Source: CAD feature listing. Evaluate the final solid. Frame: model axes, mm. Give positions to 0.01 mm unless a question says otherwise; leave off trailing zeros. Order: outer loops, then holes, each group sorted by start corner. A loop starts at its lowest first (then second) coordinate and runs counter-clockwise, first axis right, second up. Notation, with made-up numbers: (24.5, 85.5) -> (71.5, 85.5) arc R20 cw to (71.5, 93.5) -> close; hole circle Ø5 at (-34.5, -15.5). An arc over 180 degrees is marked (long way). Answer in a Markdown table with one row per item.
```python
from build123d import *

# Parameters (mm, degrees)
BOSS_EXTRUDE1_DEPTH = 4
CUT_EXTRUDE1_DEPTH  = 2
SKETCH3_R           = 11
CUT_EXTRUDE2_DEPTH  = 154.125626546


with BuildPart() as part:
    # Sketch1 → Boss-Extrude1 (new body)
    with BuildSketch(Plane.XY):
        Polygon((0, -108.239220029), (76.536686473, -76.536686473), (108.239220029, 0), (76.536686473, 76.536686473), (0, 108.239220029), (-76.536686473, 76.536686473), (-108.239220029, 0), (-76.536686473, -76.536686473), align=None)
    extrude(amount=BOSS_EXTRUDE1_DEPTH)

    # Sketch2 → Cut-Extrude1 (cut)
    with BuildSketch(Plane.XY.offset(4)):
        Polygon((-10.598200902, -12.520690706), (-1.359405577, -16.347525029), (10.598200902, 12.520690706), (1.359405577, 16.347525029), align=None)
    extrude(amount=-CUT_EXTRUDE1_DEPTH, mode=Mode.SUBTRACT)

    # Sketch3 → Cut-Extrude2 (cut, through all)
    with BuildSketch(Plane.XY.offset(4)):
        with Locations((-22.123573238, -53.411030559)):
            Circle(SKETCH3_R)
        with Locations((22.123573238, 53.411030559)):
            Circle(SKETCH3_R)
    extrude(amount=-CUT_EXTRUDE2_DEPTH, mode=Mode.SUBTRACT)


solid = part.part
```
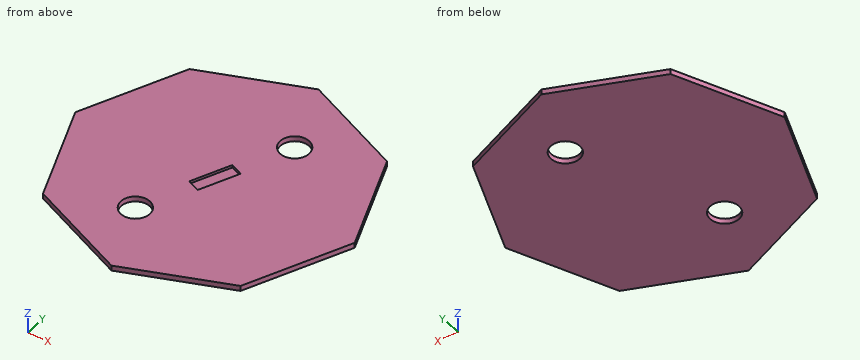
(1) First-contact query: pin 1 Ø6.5 at (x, y) = (2, 1) entering from +Z; pin 2 Ø1.5 at (y, z) = (84, 1) entering from +X; pin 3 Ø1.5 at (y, z) = (86.5, 1) entering from -X. Flat tips, straight axial feed; report the tip coordinate or a pass-through.
A:
| item | result |
|---|---|
| pin 1 | stops at z = 2 |
| pin 2 | stops at x = 60.33 |
| pin 3 | stops at x = -54.29 |
(2) Section query D-D (x = 18). Return the cut outline in (y, z), plus the area to 3 significant figures.
A:
| item | result |
|---|---|
| outline | (-100.78, 0) -> (43.21, 0) -> (43.21, 4) -> (-100.78, 4) -> close; (63.61, 0) -> (100.78, 0) -> (100.78, 4) -> (63.61, 4) -> close |
| area | 725 mm^2 |
(3) Section query A-A (x = -27.5). Return the cut outline in (y, z), plus the area to 3 significant figures.
A:
| item | result |
|---|---|
| outline | (-96.85, 0) -> (-63.01, 0) -> (-63.01, 4) -> (-96.85, 4) -> close; (-43.81, 0) -> (96.85, 0) -> (96.85, 4) -> (-43.81, 4) -> close |
| area | 698 mm^2 |
(4) Ray query, probe 1 along Y at (x, z) = (3.5, 3.4); probe 2 along Y at (x, z) = (23.5, 0.5); probe 3 along X at (y, z) = (47.5, 1.6). Return the intervals inside material, ascending.
A:
| item | result |
|---|---|
| probe 1 | y = -106.79 to -4.62, 15.46 to 106.79 |
| probe 2 | y = -98.51 to 42.5, 64.32 to 98.51 |
| probe 3 | x = -88.56 to 12.85, 31.4 to 88.56 |
(5) Section query B-B (z = 3.2). Return the cut outline in (x, y), plus the area to 3 significant figures.
A:
| item | result |
|---|---|
| outline | (-108.24, 0) -> (-76.54, -76.54) -> (0, -108.24) -> (76.54, -76.54) -> (108.24, 0) -> (76.54, 76.54) -> (0, 108.24) -> (-76.54, 76.54) -> close; hole circle Ø22 at (-22.12, -53.41); hole (-10.6, -12.52) -> (-1.36, -16.35) -> (10.6, 12.52) -> (1.36, 16.35) -> close; hole circle Ø22 at (22.12, 53.41) |
| area | 32,100 mm^2 |
(6) Section query C-C (y = 8). Return the cut outline in (x, z), plus the area to 3 significant figures.
A:
| item | result |
|---|---|
| outline | (-104.93, 0) -> (104.93, 0) -> (104.93, 4) -> (8.73, 4) -> (8.73, 2) -> (-2.1, 2) -> (-2.1, 4) -> (-104.93, 4) -> close |
| area | 818 mm^2 |
